Geometry check sheet. Reference: the model listing, model coordinates, mm. Face numbers are marked on the shaded views. A direction names the side the tool comes from. Give positions to 0.01 mm unless a question says otherwise; leave off trailing zeros. Write each loop counter-clockwise with the first axis right and the second up, starting at its lowest first coordinate (ties: lowest second). Pieces come first, ordered by that corner, then holes.
(1) Mould release check, pull along X, two halves, no side actions. Record for the marked faces 1, 2 and 3: +X half, -X half, draft (parallel to the pull), parting line (faces both ways), or undercut.
(2) Cross-section at A-A (x = 11). Record the boundary of the cut face in (y, z), and give its area (3 significant figures).
(3) Thickness scan on line 1 along Z through (x, y) = (5.5, -15.5); line 2 along X through (y, z) = (-22, 15); line 3 along Y through (x, z) = (-1, 28). Record the ranges inside material, lowest first.
(4) Depth check by flat-ended pin: P1, Ø4, axis at x = 8, z = 35.5, coming from the +Y side; P2, Ø8, axis at x = 14.5, y = -16, coming from the +Z side; P3, Ø1.5, axis at y = -10.5, z = 3.5, coming from the -X side; P4, Ø5, axis at x = -8, z = 11.5, coming from the +Y side. Enter the tip coordinate at first touch or a pass-through.
(5) Cross-section at B-B (y = -12.75). Record the boundary of the cut face in (x, z).
(6) Cross-section at D-D (x = 2). Record the boundary of the cut face in (y, z).
(7) Tool access check on the marked faces 4, 5, 6, 7 and 8. Record the directions out of +Z, -Z, +X, -X, +Y, -Y that give a thin tool (end or side, any length) a straight path to the whole face; none if there is none.
(8) Cross-section at C-C (z = 25.5). Record the boundary of the cut face in (x, y).
```python
from build123d import *

# Parameters (mm, degrees)
EXTRUDE_1_DEPTH      = 3
EXTRUDE_1_DEPTH_BACK = 2
SKETCH_2_R           = 2
EXTRUDE_2_DEPTH      = 3
FILLET_1_R           = 2
CHAMFER_1_SIZE2      = 10.001839768
CHAMFER_1_SIZE       = 10
FILLET_2_R           = 2


with BuildPart() as part:
    # 草图1 → 凸台-拉伸1 (new body, two sides)
    with BuildSketch(Plane.XY) as extrude_1_sk:
        with BuildLine():
            ThreePointArc((-6.1689615, -8.116064678), (0.566562607, -13.023133247), (8.717166108, -14.759298421))
            Line((8.717166108, -14.759298421), (17.541649585, -14.759298421))
            ThreePointArc((17.541649585, -14.759298421), (19.662969929, -15.637978077), (20.541649585, -17.759298421))
            Line((20.541649585, -17.759298421), (20.541649585, -21.259298421))
            Line((20.541649585, -21.259298421), (-5.458350415, -21.259298421))
            Line((-5.458350415, -21.259298421), (-5.458350415, -21.060154535))
            ThreePointArc((-5.458350415, -21.060154535), (-6.052483902, -20.201263808), (-7.093271049, -20.287577169))
            ThreePointArc((-7.093271049, -20.287577169), (-20.884089955, -13.119444375), (-6.1689615, -8.116064678))
        make_face()
        with BuildLine():
            ThreePointArc((-12.458350415, -17.759298421), (-8.458350415, -13.759298421), (-12.458350415, -9.759298421))
            ThreePointArc((-12.458350415, -9.759298421), (-16.458350415, -13.759298421), (-12.458350415, -17.759298421))
        make_face(mode=Mode.SUBTRACT)
        Polygon((18.541649585, -23.259298421), (-3.458350415, -23.259298421), (-5.458350415, -23.259298421), (-5.458350415, -21.259298421), (20.541649585, -21.259298421), (20.541649585, -23.259298421), align=None)
    extrude(amount=EXTRUDE_1_DEPTH)
    extrude(extrude_1_sk.sketch, amount=-EXTRUDE_1_DEPTH_BACK)

    # 草图2 → 凸台-拉伸2 (add)
    with BuildSketch(Plane.XZ.offset(23.259298421)):
        Polygon((20.541649585, 46.004782855), (-5.458350415, 46.000000778), (-5.458350415, 2), (-5.458350415, -2), (20.541649585, -2), align=None)
        with Locations((10.541649585, 40.750439451)):
            Circle(SKETCH_2_R, mode=Mode.SUBTRACT)
        with Locations((10.541649585, 10.750439451)):
            Circle(SKETCH_2_R, mode=Mode.SUBTRACT)
    extrude(amount=-EXTRUDE_2_DEPTH)

    # 圆角1
    fillet_1_edges = [part.edges().sort_by_distance(p)[0] for p in [
        (7.541649585, -23.259298421, -2),
    ]]
    fillet(fillet_1_edges, radius=FILLET_1_R)

    # 倒角1
    chamfer_1_edges = [part.edges().sort_by_distance(p)[0] for p in [
        (-5.458350415, -21.759298421, 46.000000778),
    ]]
    chamfer(chamfer_1_edges, length=CHAMFER_1_SIZE, length2=CHAMFER_1_SIZE2)

    # 圆角2
    fillet_2_edges = [part.edges().sort_by_distance(p)[0] for p in [
        (7.541649585, -20.259298421, 3),
    ]]
    fillet(fillet_2_edges, radius=FILLET_2_R)


solid = part.part
```
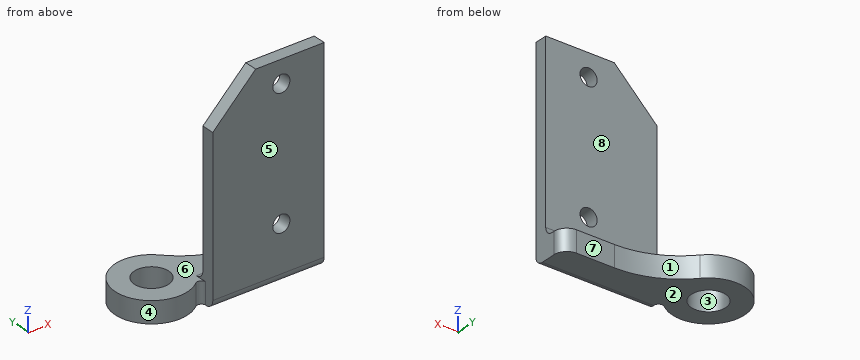
Reply:
1. face 1: +X half
1. face 2: draft
1. face 3: undercut
2. outline: (-23.26, 0) arc R2 ccw to (-21.26, -2) - (-14.76, -2) - (-14.76, 3) - (-18.26, 3) arc R2 cw to (-20.26, 5) - (-20.26, 8.8) - (-23.26, 8.8) - close; (-23.26, 12.7) - (-20.26, 12.7) - (-20.26, 38.8) - (-23.26, 38.8) - close; (-23.26, 42.7) - (-20.26, 42.7) - (-20.26, 46) - (-23.26, 46) - close
2. area: 148 mm2
3. line 1: z = -2 to 3
3. line 2: x = -5.46 to 20.54
3. line 3: y = -23.26 to -20.26
4. P1: stops at y = -20.26
4. P2: stops at z = 4.02
4. P3: stops at x = -20.47
4. P4: passes through
5. outline: (-20.85, -2) - (-16.33, -2) - (-16.33, 3) - (-20.85, 3) - close; (-8.59, -2) - (-0.02, -2) - (-0.02, 3) - (-8.59, 3) - close
6. outline: (-23.26, 0) arc R2 ccw to (-21.26, -2) - (-13.6, -2) - (-13.6, 3) - (-18.26, 3) arc R2 cw to (-20.26, 5) - (-20.26, 43.46) - (-23.26, 43.46) - close
7. face 4: +Z, -Z
7. face 5: +Z, -Z, +X, -X, -Y
7. face 6: +Z, -X, +Y
7. face 7: +Z, -Z, +X, +Y
7. face 8: +Z, +X, -X, +Y
8. outline: (-5.46, -23.26) - (20.54, -23.26) - (20.54, -20.26) - (-5.46, -20.26) - close
